```python
from build123d import *

# Parameters (mm, degrees)
F0_R     = 53.3741720423
F1_DEPTH = 12.7
F2_SIZE  = 5.08
F3_DEPTH = 2.54


# Not quite as in the source:
# - a fillet or chamfer that OpenCascade refuses, or shapes differently, is made with other operations: its cross-section is extruded or revolved along the edge and cut away or added


with BuildPart() as f1:
    # F0 (on Top) → F1 (new body)
    with BuildSketch(Plane.XY):
        with Locations((18.2692110538, -6.3352882862)):
            Circle(F0_R)
    extrude(amount=F1_DEPTH)

    # F2
    f2_edges = [f1.edges().sort_by_distance(p)[0] for p in [
        (-35.104961, -6.335288, 12.7),
        (-35.104961, -6.335288, 0),
        (71.643383, -6.335288, 6.35),
    ]]
    chamfer(f2_edges, length=F2_SIZE)

    # F3 (add): a face of the model
    f3_faces = [f1.faces().sort_by_distance(p)[0] for p in [
        (18.2692110538, -6.3352882862, 12.7),
    ]]
    extrude(f3_faces, amount=F3_DEPTH)

    # F4: fillet of radius 5.08 on 1 edges, made by hand

    # F4_s1 → F4_t2 (revolve, cut)
    with BuildSketch(Plane.XZ.offset(6.3352882862)):
        with BuildLine():
            ThreePointArc((66.5633830961, 12.7), (64.7039740449, 14.5594090512), (62.1639740449, 15.24))
            Line((62.1639740449, 15.24), (62.1639740449, 15.3416))
            Line((62.1639740449, 15.3416), (66.5633830961, 15.3416))
            Line((66.5633830961, 15.3416), (66.6649830961, 15.24))
            ThreePointArc((66.6649830961, 15.24), (66.6649830961, 13.97), (66.6513712772, 12.7508))
            Line((66.6513712772, 12.7508), (66.5633830961, 12.7))
        make_face()
    revolve(axis=Axis((18.2692110538, -6.3352882862, 15.24), (0, 0, 1)), mode=Mode.SUBTRACT)


solid = f1.part
```
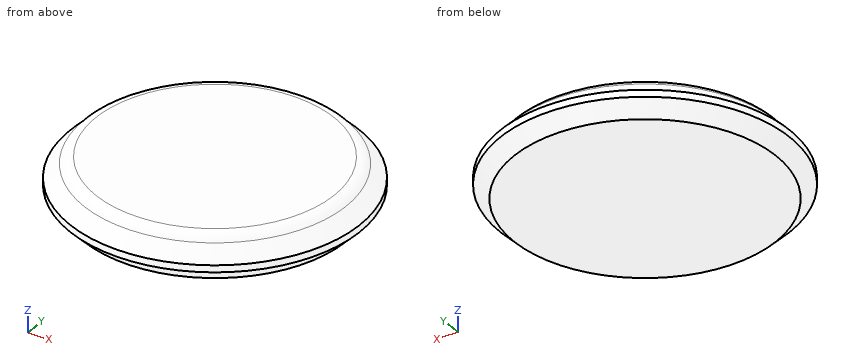
The listing builds one solid part. Answer for the finished solid, in the listing's coordinates (mm). Coordinates: 2 decimals unless noted, no trailing zeros. Order: outer loops, then holes, each group sorted by start corner. A loop starts at its lowest first (then second) coordinate and runs counter-clockwise, first axis right, second up. Notation, with made-up numbers: M 71.5,-24.5 L 89.5,-24.5 A24 ccw 89.5,-14.5 Z; hole C -35,25.5 d1. An arc over 180 degrees is marked long. Answer as a JSON object with one key per item and string values. Group by question number.
1. Flat-ended cylindrical pins translate along their axes: P1, Ø8, axis at y = -26.5, z = 7, coming from the +X side; P2, Ø6, axis at x = 24, z = 13.5, coming from the -Y side; P3, Ø2, axis at y = -34, z = 12.5, coming from the -X side. Find the tip coordinate at first contact, or state that the pin passes through.
2. Section A-A on z = 1.5 is taken. Write down the section's boundary in (x, y), then the cut area to 3 significant figures.
3. Straight lines are drawn through the part: line 1 (X direction, y = 10, z = 4.5); line 2 (Y direction, x = 9, z = 2.75); line 3 (Y direction, x = -23, z = 1.75). For each, find the intervals that lie inside material, in ascending order.
Values follow:
{
 "1": {"P1": "x = 69.14", "P2": "y = -56.52", "P3": "x = -22.94"},
 "2": {"outline": "C 18.27,-6.34 d99.59", "area": "7,790 mm2"},
 "3": {"line 1": "-31.93 to 68.47", "line 2": "-56.53 to 43.86", "line 3": "-34.64 to 21.97"}
}
